```python
from build123d import *

# Parameters (mm, degrees)
F1_DEPTH = 38
F2_R     = 0.8
F3_R     = 1
F4_SIZE  = 0.5


with BuildPart() as f1:
    # F0 (on Top) → F1 (new body)
    with BuildSketch(Plane.XY):
        with BuildLine():
            Line((-4.05, -6), (4.05, -6))
            Line((4.05, -6), (4.05, -3.579106))
            ThreePointArc((4.05, -3.579106), (-2.05, 0), (4.05, 3.579106))
            Line((4.05, 3.579106), (4.05, 6))
            Line((4.05, 6), (-4.05, 6))
            Line((-4.05, 6), (-4.05, -6))
        make_face()
    extrude(amount=F1_DEPTH)

    # F2
    f2_edges = [f1.edges().sort_by_distance(p)[0] for p in [
        (4.05, 3.579106, 19),
        (4.05, -3.579106, 19),
    ]]
    fillet(f2_edges, radius=F2_R)

    # F3
    f3_edges = [f1.edges().sort_by_distance(p)[0] for p in [
        (4.05, 6, 19),
        (4.05, -6, 19),
        (-4.05, -6, 19),
        (-4.05, 6, 19),
    ]]
    fillet(f3_edges, radius=F3_R)

    # F4
    f4_edges = [f1.edges().sort_by_distance(p)[0] for p in [
        (-2.05, 0, 38),
        (-2.05, 0, 0),
    ]]
    chamfer(f4_edges, length=F4_SIZE)


solid = f1.part
```
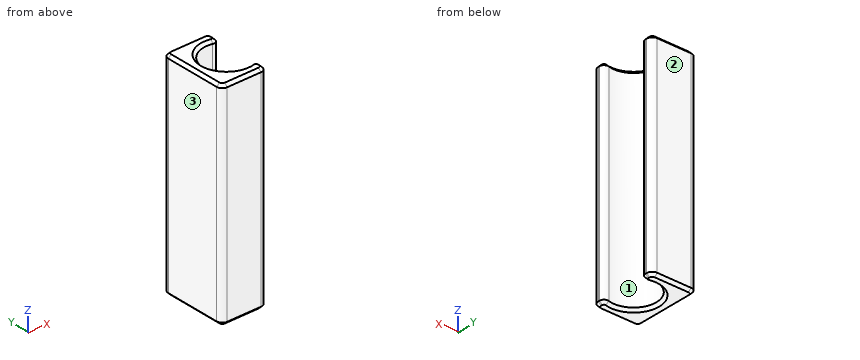
Could you check a few things on this model? Use its own coordinates, in mm. Face numbers are marked on the shaded views. Round coordinates to 2 decimals unless told otherwise and drop trailing zeros. Order: outer loops, then holes, each group sorted by start corner. A loop starts at its lowest first (then second) coordinate and runs counter-clockwise, first axis right, second up. Notation, with made-up numbers: M -32.75,-19 L 24.25,-19 A27 cw 24.25,17 Z; hole C 35.5,77 d5. An arc over 180 degrees is marked long. One line per question, with ' | ' between items. Start each with the question number.
(1) Suppose I cut it at A-A on x = 2.05. List the corners of the cut face in (y, z) for me.
(2) For P1, Ø1, axis at x = 0, y = 0.5, coming from the -Z side, with a flat end and sliding along its axis, tell me the tip position at first contact or that it passes through.
(3) Suppose I cut it at B-B on y = 0. List the corners of the cut face in (x, z) for me, then the cut area to 3 significant figures.
(4) Suppose I cut it at C-C on z = 35. List the corners of the cut face in (x, y) for me.
(5) Please list where these lines run through material, in increasing order: line 1 along Y through (x, z) = (2.05, 15.5); line 2 along Y through (x, z) = (3, 7); line 3 along X through (y, z) = (-0.25, 36.5).
(6) Thinking about a two-plate mould opening in X: for the marked faces 1, 2 and 3, which applies, +X half, -X half, draft (parallel to the pull), parting line (faces both ways), or undercut?
Geometry results:
1) outline: M -6,0.5 L -5.5,0 L -4.6,0 L -4.1,0.5 L -4.1,37.5 L -4.6,38 L -5.5,38 L -6,37.5 Z; M 4.1,0.5 L 4.6,0 L 5.5,0 L 6,0.5 L 6,37.5 L 5.5,38 L 4.6,38 L 4.1,37.5 Z
2) P1: through
3) outline: M -4.05,0.5 L -3.55,0 L -2.55,0 L -2.05,0.5 L -2.05,37.5 L -2.55,38 L -3.55,38 L -4.05,37.5 Z | area: 75.5 mm²
4) outline: M -4.05,-5 A1 ccw -3.05,-6 L 3.05,-6 A1 ccw 4.05,-5 L 4.05,-4.75 A0.8 ccw 3.05,-3.98 A4.1 cw long 3.05,3.98 A0.8 ccw 4.05,4.75 L 4.05,5 A1 ccw 3.05,6 L -3.05,6 A1 ccw -4.05,5 Z
5) line 1: -6 to -4.1, 4.1 to 6 | line 2: -6 to -3.99, 3.99 to 6 | line 3: -4.05 to -2.04
6) face 1: undercut | face 2: draft | face 3: -X half
